```python
from build123d import *

# Parameters (mm, degrees)
SKETCH_1_W      = 13
SKETCH_1_H      = 9
EXTRUDE_1_DEPTH = 7
SKETCH_2_R      = 2.85
EXTRUDE_2_DEPTH = 7


with BuildPart() as part:
    # 草图1 → 凸台-拉伸1 (new body)
    with BuildSketch(Plane.XY):
        Rectangle(SKETCH_1_W, SKETCH_1_H)
    extrude(amount=EXTRUDE_1_DEPTH)

    # 草图2 → 凸台-拉伸2 (add)
    with BuildSketch(Plane(origin=(0, 4.5, 0), x_dir=(1, 0, 0), z_dir=(0, 1, 0))):
        with Locations(Location((0, -3.5, 0), (0, 0, 180))):
            Circle(SKETCH_2_R)
    extrude(amount=EXTRUDE_2_DEPTH)

    # 草图3 → 旋转1 (revolve)
    with BuildSketch(Plane(origin=(0, 0, 0), x_dir=(0, 0, -1), z_dir=(1, 0, 0)), mode=Mode.PRIVATE) as revolve_1_sk:
        with BuildLine():
            Line((-3.5, 11.5), (-4.8, 11.5))
            Line((-4.8, 11.5), (-5, 21))
            ThreePointArc((-5, 21), (-4.560660172, 22.060660172), (-3.5, 22.5))
            Line((-3.5, 22.5), (-3.5, 11.5))
        make_face()
    revolve(revolve_1_sk.sketch.rotate(Axis((0, 11.5, 3.5), (0, 1, 0)), 180), axis=Axis((0, 11.5, 3.5), (0, 1, 0)))


solid = part.part
```
Can you work these out from the model? Positions are in its coordinate system, mm. A direction names the side the tool comes from. Round coordinates to 2 decimals unless told otherwise and drop trailing zeros. Loops run counter-clockwise (first coordinate to the right, second up) from the corner with the lowest first, then second, coordinate; pieces in that order, holes last. Notation, with made-up numbers: M 37.5,-31.5 L 67.5,-31.5 A25 ccw 67.5,0.5 Z; hole C 7,22 d11. An arc over 180 degrees is marked long. Write item = value, one per line. Start each with the question number.
(1) I need wall thicknesses on line 1 along Y through (x, z) = (3, 6.25); line 2 along Y through (x, z) = (-2.5, 3.75); line 3 along Z through (x, y) = (-1.25, 7.25). Which ranges of each line are inside material? Lowest first, please.
(2) Suppose I cut it at A-A on z = 3.5. Write out the boundary of the cut face in (x, y).
(3) Suppose I cut it at B-B on x = 0. Write out the boundary of the cut face in (y, z).
(4) I'm going to push flat-ended pins straight in: P1, Ø1.7, axis at x = 1, z = 4, coming from the +Y side; P2, Ø2, axis at x = -1, z = 2.5, coming from the +Y side; P3, Ø6, axis at x = 1, y = 8, coming from the -Z side. Where does each tip first touch, or does it pass through?
(5) If we mould it in two halves opening along Y, with no side actions, what happens to faces 1 (the face through (0, -4.5, 3)), 2 (the face through (0.853, 16.316, 4.612)), 3 (the face through (-6.5, 0, 3))? For each: released by +Y, released by -Y, zero draft, split by the parting line, or undercut.
(6) Suppose I cut it at C-C on y = 7. Write out the boundary of the cut face in (x, z), plus the area to 3 significant figures.
(7) Which directions (+Z, -Z, +X, -X, +Y, -Y) give clear straight access to the entire face, cutting with the end or side of a thin tool? Please do faces 4 (the face through (-1, 11.5, 2)), 5 (the face through (0.371, 7.951, 6.326)), 6 (the face through (0, 0, 0)).
(8) Suppose I cut it at D-D on z = 5.25. Write out the boundary of the cut face in (x, y), plus the area to 3 significant figures.
Answer block:
q1.line_1 = -4.5 to 4.5
q1.line_2 = -4.5 to 11.5
q1.line_3 = 0.94 to 6.06
q2.outline = M -6.5,-4.5 L 6.5,-4.5 L 6.5,4.5 L 2.85,4.5 L 2.85,11.5 L 1.3,11.5 L 1.5,21 A1.5 ccw -1.5,21 L -1.3,11.5 L -2.85,11.5 L -2.85,4.5 L -6.5,4.5 Z
q3.outline = M -4.5,0 L 4.5,0 L 4.5,0.65 L 11.5,0.65 L 11.5,2.2 L 21,2 A1.5 ccw 21,5 L 11.5,4.8 L 11.5,6.35 L 4.5,6.35 L 4.5,7 L -4.5,7 Z
q4.P1 = 22.48
q4.P2 = 22.44
q4.P3 = 0.65
q5.face_1 = released by -Y
q5.face_2 = undercut
q5.face_3 = zero draft
q6.outline = C 0,3.5 d5.7
q6.area = 25.5 mm²
q7.face_4 = none
q7.face_5 = +Y
q7.face_6 = -Z, +X, -X, +Y, -Y
q8.outline = M -6.5,-4.5 L 6.5,-4.5 L 6.5,4.5 L 2.25,4.5 L 2.25,11.5 L -2.25,11.5 L -2.25,4.5 L -6.5,4.5 Z
q8.area = 148 mm²
